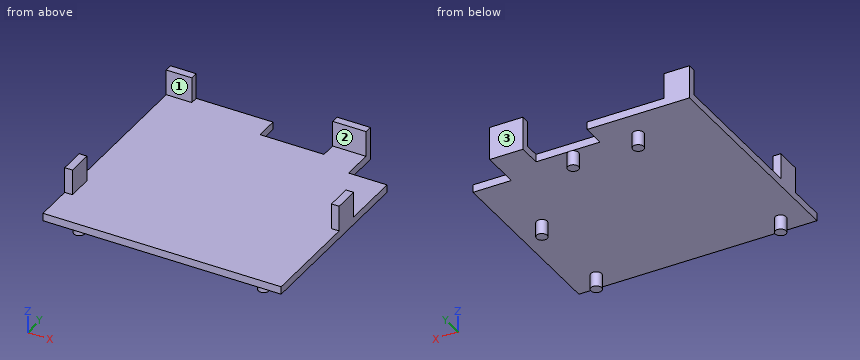
Autodesk Inventor part; units mm, degrees
ref_plane "YZ Plane" through (0, 0, 0) normal (1, 0, 0) x (0, 1, 0)
ref_plane "XZ Plane" through (0, 0, 0) normal (0, 1, 0) x (-1, 0, 0)
ref_plane "XY Plane" through (0, 0, 0) normal (0, 0, 1) x (1, 0, 0)
sketch "Esquisse1" plane through (0, 0, 0) normal (0, 1, 0) x (-1, 0, 0)
  line L0 (-46.5, 50) -> (46.5, 50)
  line L1 (46.5, 50) -> (46.5, -50)
  line L2 (46.5, -50) -> (-46.5, -50)
  line L3 (-46.5, -50) -> (-46.5, 50)
  line L4 (-46.5, 50) -> (46.5, -50) construction
  line L5 (46.5, 50) -> (-46.5, -50) construction
  point P0 (0, 0)
  dimension "d0" = 100
  dimension "d1" = 93
extrude "Extrusion1" add sketch "Esquisse1" along normal blind 88
sketch "Esquisse2" plane through (0, 0, 0) normal (0, -1, 0) x (1, 0, 0)
  line L0 (-43.5, 47) -> (43.5, 47)
  line L1 (43.5, 47) -> (43.5, -47)
  line L2 (43.5, -47) -> (-43.5, -47)
  line L3 (-43.5, -47) -> (-43.5, 47)
  line L4 (-43.5, 47) -> (43.5, -47) construction
  line L5 (43.5, 47) -> (-43.5, -47) construction
  line L6 (46.5, 50) -> (46.5, -50)
  line L7 (-46.5, 50) -> (46.5, 50)
  point P0 (0, 0)
  dimension "d4" = 3
  dimension "d5" = 3
extrude "Extrusion2" cut sketch "Esquisse2" against normal blind 85
sketch "Esquisse3" plane through (-46.5, 0, 50) normal (0, 0, 1) x (1, 0, 0)
  line L0 (0, 88) -> (93, 88)
  line L1 (93, 88) -> (78, 88)
  line L2 (78, 88) -> (78, 73)
  line L3 (78, 73) -> (93, 73)
  line L4 (93, 73) -> (93, 88)
  point P0 (46.5, 0)
  dimension "d8" = 15
  dimension "d9" = 15
extrude "Extrusion3" cut sketch "Esquisse3" against normal up to surface (100 mm away)
sketch "Esquisse4" plane through (-46.5, 0, 50) normal (0, 0, 1) x (1, 0, 0)
  circle A0 centre (73, 68) radius 1.75
  circle A1 centre (33, 68) radius 1.75
  circle A2 centre (73, 30) radius 1.75
  circle A3 centre (33, 30) radius 1.75
  line L0 (93, 0) -> (93, 73)
  line L1 (0, 88) -> (78, 88)
  point P0 (46.5, 0)
  dimension "d12" = 40
  dimension "d13" = 3.5
  dimension "d14" = 3.5
  dimension "d15" = 3.5
  dimension "d16" = 3.5
  dimension "d17" = 40
  dimension "d18" = 0
  dimension "d19" = 0
  dimension "d20" = 38
  dimension "d21" = 20
  dimension "d22" = 20
  dimension "d23" = 0
extrude "Extrusion4" cut sketch "Esquisse4" against normal up to surface (3 mm away)
sketch "Esquisse5" plane through (46.5, 0, -50) normal (0, 0, -1) x (-1, 0, 0)
  circle A0 centre (66.8, 77) radius 2.1
  circle A1 centre (41.4, 77) radius 2.1
  circle A2 centre (11, 44.9) radius 2.1
  circle A3 centre (11, 7.4) radius 2.1
  line L0 (0, 0) -> (0, 73)
  line L1 (15, 88) -> (93, 88)
  line L2 (15, 88) -> (15, 73)
  line L3 (15, 73) -> (0, 73)
  circle A4 centre (83, 7.4) radius 2.1
  line L4 (93, 0) -> (93, 88)
  point P0 (46.5, 0)
  dimension "d26" = 4.2
  dimension "d27" = 4.2
  dimension "d28" = 4.2
  dimension "d29" = 4.2
  dimension "d30" = 11
  dimension "d31" = 0
  dimension "d32" = 11
  dimension "d33" = 0
  dimension "d34" = 37.5
  dimension "d35" = 25.4
  dimension "d36" = 26.4
  dimension "d37" = 28.1
  dimension "d38" = 4.2
  dimension "d39" = 0
  dimension "d40" = 10
extrude "Extrusion5" add sketch "Esquisse5" along normal blind 5.7
sketch "Esquisse6" plane through (-36.5, 7.4, -55.7) normal (0, 0, -1) x (-1, 0, 0)
  point P0 (-36.5, -7.4)
sketch "Esquisse7" plane through (-46.5, 0, 50) normal (0, 0, 1) x (1, 0, 0)
  line L0 (0, 88) -> (78, 88)
  line L1 (65, 88) -> (40, 88)
  line L2 (40, 88) -> (40, 79)
  line L3 (40, 79) -> (65, 79)
  line L4 (65, 79) -> (65, 88)
  line L5 (78, 73) -> (78, 88)
  point P0 (46.5, 0)
  point P1 (78, 80.5)
  point P2 (65, 83.5)
  dimension "d43" = 25
  dimension "d44" = 13
  dimension "d45" = 9
extrude "Extrusion6" cut sketch "Esquisse7" against normal up to surface (100 mm away)
sketch "Esquisse8" plane through (-46.5, 0, 50) normal (0, 0, 1) x (1, 0, 0)
  line L0 (0, 0) -> (0, 88)
  line L1 (0, 0) -> (94.9117, 0)
  line L2 (94.9117, 0) -> (94.9117, 90.3204)
  line L3 (94.9117, 90.3204) -> (0, 90.3204)
  line L4 (0, 90.3204) -> (0, 0)
  point P0 (46.5, 0)
extrude "Extrusion7" cut sketch "Esquisse8" against normal up to surface (97 mm away)
sketch "Esquisse9" plane through (-46.5, 0, -47) normal (0, 0, 1) x (1, 0, 0)
  line L0 (78, 88) -> (65, 88)
  line L1 (78, 88) -> (78, 73)
  line L2 (65, 88) -> (78, 88)
  line L3 (78, 88) -> (78, 85)
  line L4 (78, 85) -> (65, 85)
  line L5 (65, 85) -> (65, 88)
  line L6 (0, 88) -> (10, 88)
  line L7 (10, 88) -> (10, 85)
  line L8 (10, 85) -> (0, 85)
  line L9 (0, 85) -> (0, 88)
  line L10 (0, 0) -> (0, 88)
  line L11 (0, 15) -> (3, 15)
  line L12 (3, 15) -> (3, 25)
  line L13 (3, 25) -> (0, 25)
  line L14 (0, 25) -> (0, 15)
  line L15 (93, 0) -> (0, 0)
  line L16 (93, 73) -> (93, 0)
  line L17 (93, 50) -> (90, 50)
  line L18 (90, 50) -> (90, 40)
  line L19 (90, 40) -> (93, 40)
  line L20 (93, 40) -> (93, 50)
  point P0 (46.5, 0)
  point P1 (0, 25)
  dimension "d50" = 3
  dimension "d51" = 3
  dimension "d52" = 10
  dimension "d53" = 15
  dimension "d54" = 10
  dimension "d55" = 3
  dimension "d56" = 40
  dimension "d57" = 10
  dimension "d58" = 3
extrude "Extrusion8" add sketch "Esquisse9" along normal blind 10
properties part number "support_imu_Impression 3D"
Geometry: final body of the model. Coordinates: model frame, mm. Face numbers are marked on the shaded views. Round coordinates to 2 decimals unless told otherwise and drop trailing zeros. Loops run counter-clockwise (first coordinate to the right, second up) from the corner with the lowest first, then second, coordinate; pieces in that order, holes last.
Q1. Pin query (flat end, axial travel): P1, Ø11, axis at x = 22, z = -40, coming from the -Y side; P2, Ø0.9, axis at x = 45, z = -41, coming from the -Y side; P3, Ø0.9, axis at x = 37.5, z = -48, coming from the +Y side; P4, Ø5, axis at x = -32.5, z = -43, coming from the -Y side. Return the tip coordinate at first contact, or that it passes through.
Q2. Pull-direction query (Y, two-part tool) for the marked faces 1, 2 and 3; classes: released by +Y, released by -Y, zero draft, split by the parting line, or undercut.
Q3. Section C-C on x = -20.3. Return loops of the section in (y, z).
Q4. Section D-D on y = 48.5. Return loops of the section in (x, z).
Q5. Section A-A on z = -44. Return loops of the section in (x, y).
Q6. Material intervals for L1, parallel to Z at x = -34, y = 25; L2, parallel to X at y = 16.5, z = -37.75; L3, parallel to Y at x = -40.5, z = -42, sorted ascending.
Q7. Section B-B on y = 7.4. Return loops of the section in (x, z).
Evaluation:
1. P1: stops at y = 85
1. P2: stops at y = 40
1. P3: stops at y = 73
1. P4: passes through
2. face 1: undercut
2. face 2: released by -Y
2. face 3: released by +Y
3. outline: (0, -50) - (74.9, -50) - (74.9, -55.7) - (79.1, -55.7) - (79.1, -50) - (88, -50) - (88, -47) - (0, -47) - close
4. outline: (-46.5, -50) - (46.5, -50) - (46.5, -37) - (43.5, -37) - (43.5, -47) - (-46.5, -47) - close
5. outline: (-46.5, 15) - (-43.5, 15) - (-43.5, 25) - (-46.5, 25) - close; (-46.5, 85) - (-36.5, 85) - (-36.5, 88) - (-46.5, 88) - close; (18.5, 85) - (31.5, 85) - (31.5, 88) - (18.5, 88) - close; (43.5, 40) - (46.5, 40) - (46.5, 50) - (43.5, 50) - close
6. L1: z = -50 to -47
6. L2: x = -46.5 to -43.5
6. L3: y = 85 to 88
7. outline: (-46.5, -50) - (-38.6, -50) - (-38.6, -55.7) - (-34.4, -55.7) - (-34.4, -50) - (33.4, -50) - (33.4, -55.7) - (37.6, -55.7) - (37.6, -50) - (46.5, -50) - (46.5, -47) - (-46.5, -47) - close
